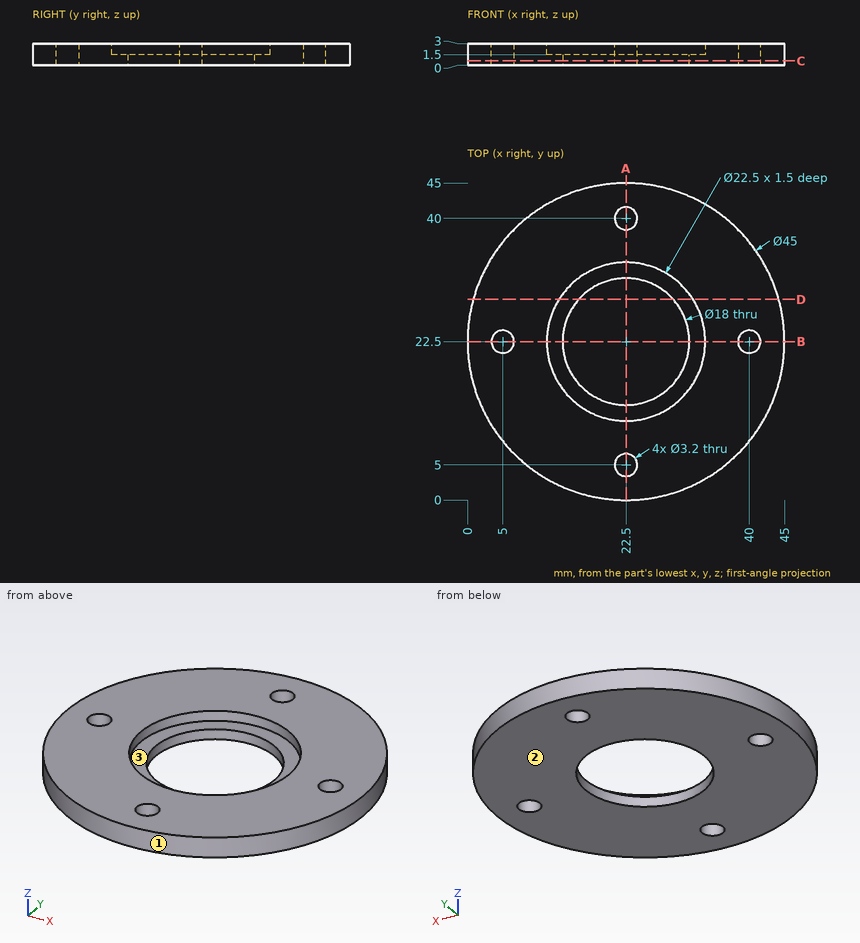
Print and shaded views of the part. All mm, measured from the part's lowest x, y and z. Round coordinates to 2 decimals unless told otherwise and drop trailing zeros. Write each loop counter-clockwise with the first axis right and the second up, starting at its lowest first coordinate (ties: lowest second). Pieces come first, ordered by that corner, then holes.
(1) Probe line 1 along Y through (x, z) = (22, 1.85); line 2 along Z through (x, y) = (16.5, 31.5); line 3 along Y through (x, z) = (40, 2.35). List the from-to ranges inside material, lowest first.
(2) Slice it at A-A, the plane x = 22.5. Write the cut outline in (y, z), and give its area (4 significant figures).
(3) Drop flat-ended pins along their axis: P1, Ø7, axis at x = 25.5, y = 27.5, coming from the +Z side; P2, Ø1.5, axis at x = 9.5, z = 2.5, coming from the -Y side. Give the stop position or say it passes through.
(4) Slice it at D-D, the plane y = 28.5. Write the cut outline in (x, z), and give its area (3 significant figures).
(5) Mould opens along Y. For the marked faces 1, 2 and 3 say: pulls with the +Y half, pulls with the -Y half, needs draft (parallel to the pull), parting line crosses it, or undercut.
(6) Slice it at C-C, the plane z = 0.6. Write the cut outline in (x, y), and give its area (3 significant figures).
From the geometry:
1. line 1: y = 0.01 to 3.48, 6.52 to 11.26, 33.74 to 38.48, 41.52 to 44.99
1. line 2: z = 0 to 1.5
1. line 3: y = 8.36 to 20.9, 24.1 to 36.64
2. outline: (0, 0) - (3.4, 0) - (3.4, 3) - (0, 3) - close; (6.6, 0) - (13.5, 0) - (13.5, 1.5) - (11.25, 1.5) - (11.25, 3) - (6.6, 3) - close; (31.5, 0) - (38.4, 0) - (38.4, 3) - (33.75, 3) - (33.75, 1.5) - (31.5, 1.5) - close; (41.6, 0) - (45, 0) - (45, 3) - (41.6, 3) - close
2. area: 55.05 mm2
3. P1: stops at z = 1.5
3. P2: stops at y = 3.63
4. outline: (0.81, 0) - (15.79, 0) - (15.79, 1.5) - (12.98, 1.5) - (12.98, 3) - (0.81, 3) - close; (29.21, 0) - (44.19, 0) - (44.19, 3) - (32.02, 3) - (32.02, 1.5) - (29.21, 1.5) - close
4. area: 81.4 mm2
5. face 1: parting line crosses it
5. face 2: needs draft
5. face 3: undercut
6. outline: circle Ø45 at (22.5, 22.5); hole circle Ø3.2 at (5, 22.5); hole circle Ø18 at (22.5, 22.5); hole circle Ø3.2 at (22.5, 5); hole circle Ø3.2 at (22.5, 40); hole circle Ø3.2 at (40, 22.5)
6. area: 1,300 mm2
